Geometry: final body of the model. Coordinates: model frame, mm. Face numbers are marked on the shaded views. Give positions to 0.01 mm unless a question says otherwise; leave off trailing zeros. Write each loop counter-clockwise with the first axis right and the second up, starting at its lowest first coordinate (ties: lowest second). Pieces come first, ordered by that corner, then holes.
Q1. Mould query, pull axis Y, two halves, no side actions, for the marked faces 1 and 2. Classes: +Y half, -Y half, draft (parallel to the pull), parting line (faces both ways), or undercut.
Q2. Line query: line 1 (X direction, y = 81.5, z = -4.55); line 2 (X direction, y = 71.5, z = -4.15); line 3 (X direction, y = 40.5, z = -3.5). Output: solid intervals per line, ascending.
Q3. Section C-C (y = 42). Return the cut outline in (x, z), plus the area to 3 significant figures.
Q4. Section B-B (z = -1.2). Return the cut outline in (x, y).
Q5. Section A-A (x = 21). Return the cut outline in (y, z), plus the area to 3 significant figures.
Q6. Pin query (flat end, axial travel): pin 1 Ø2 at (y, z) = (83, -1.5) entering from -X; pin 2 Ø2.5 at (x, z) = (28.5, -1.5) entering from +Y. Return the tip coordinate at first contact, or that it passes through.
Q7. Section D-D (x = 30). State how many separate pieces and enclosed holes the cut face has, plus the area to 3 significant figures.
from build123d import *

# Parameters (mm, degrees)
SKETCH1_W          = 60
SKETCH1_H          = 100
SKETCH1_W_2        = 20
SKETCH1_H_2        = 40
EXTRUDE1_DEPTH     = 5
FILLET2_R          = 3
SHELL2_START       = -5
SHELL2_OUTLINE_W   = 55
SHELL2_OUTLINE_H   = 95
SHELL2_OUTLINE_W_2 = 25
SHELL2_OUTLINE_H_2 = 45
SHELL2_DEPTH       = 2.5
SHELL2_START_2     = 2.5
SHELL2_2_DEPTH     = 95
SHELL2_START_3     = 2
SHELL2_3_DEPTH     = 56


with BuildPart() as part:
    # Sketch1 → Extrude1 (new body)
    with BuildSketch(Plane.XY):
        with Locations((30, 50)):
            Rectangle(SKETCH1_W, SKETCH1_H)
        with Locations((30, 50)):
            Rectangle(SKETCH1_W_2, SKETCH1_H_2, mode=Mode.SUBTRACT)
        with BuildLine():
            Line((32.5, 80), (32.5, 90))
            ThreePointArc((32.5, 90), (30, 92.5), (27.5, 90))
            Line((27.5, 90), (27.5, 80))
            ThreePointArc((27.5, 80), (30, 77.5), (32.5, 80))
        make_face(mode=Mode.SUBTRACT)
        with BuildLine():
            Line((27.5, 10), (27.5, 20))
            ThreePointArc((27.5, 20), (30, 22.5), (32.5, 20))
            Line((32.5, 20), (32.5, 10))
            ThreePointArc((32.5, 10), (30, 7.5), (27.5, 10))
        make_face(mode=Mode.SUBTRACT)
    extrude(amount=-EXTRUDE1_DEPTH)

    # Fillet2
    fillet2_edges = [part.edges().sort_by_distance(p)[0] for p in [
        (30, 100, 0),
        (60, 50, 0),
        (30, 0, 0),
        (0, 50, 0),
    ]]
    fillet(fillet2_edges, radius=FILLET2_R)

    # Shell2: read off the stored shape, not the designer's step
    # Shell2 outline → Shell2 (cut)
    with BuildSketch(Plane.XY.offset(SHELL2_START)):
        with Locations((30, 50)):
            Rectangle(SHELL2_OUTLINE_W, SHELL2_OUTLINE_H)
        with BuildLine():
            Line((25, 10), (25, 20))
            ThreePointArc((25, 20), (30, 25), (35, 20))
            Line((35, 20), (35, 10))
            ThreePointArc((35, 10), (30, 5), (25, 10))
        make_face(mode=Mode.SUBTRACT)
        with Locations((30, 50)):
            Rectangle(SHELL2_OUTLINE_W_2, SHELL2_OUTLINE_H_2, mode=Mode.SUBTRACT)
        with BuildLine():
            ThreePointArc((35, 80), (30, 75), (25, 80))
            Line((25, 80), (25, 90))
            ThreePointArc((25, 90), (30, 95), (35, 90))
            Line((35, 90), (35, 80))
        make_face(mode=Mode.SUBTRACT)
    extrude(amount=SHELL2_DEPTH, mode=Mode.SUBTRACT)

    # Shell2 2 outline → Shell2 2 (add)
    with BuildSketch(Plane(origin=(0, 0, 0), x_dir=(1, 0, 0), z_dir=(0, 1, 0)).offset(SHELL2_START_2)):
        with BuildLine():
            Line((57.5, 2.5), (57.5, 3))
            ThreePointArc((57.5, 3), (57.353553391, 2.646446609), (57, 2.5))
            Line((57, 2.5), (57.5, 2.5))
        make_face()
        with BuildLine():
            Line((2.5, 2.5), (3, 2.5))
            ThreePointArc((3, 2.5), (2.646446609, 2.646446609), (2.5, 3))
            Line((2.5, 3), (2.5, 2.5))
        make_face()
    extrude(amount=SHELL2_2_DEPTH)

    # Shell2 3 outline → Shell2 3 (add)
    with BuildSketch(Plane.YZ.offset(SHELL2_START_3)):
        with BuildLine():
            ThreePointArc((2.5, -3), (2.646446609, -2.646446609), (3, -2.5))
            Line((3, -2.5), (2.5, -2.5))
            Line((2.5, -2.5), (2.5, -3))
        make_face()
        with BuildLine():
            ThreePointArc((97, -2.5), (97.353553391, -2.646446609), (97.5, -3))
            Line((97.5, -3), (97.5, -2.5))
            Line((97.5, -2.5), (97, -2.5))
        make_face()
    extrude(amount=SHELL2_3_DEPTH)


solid = part.part
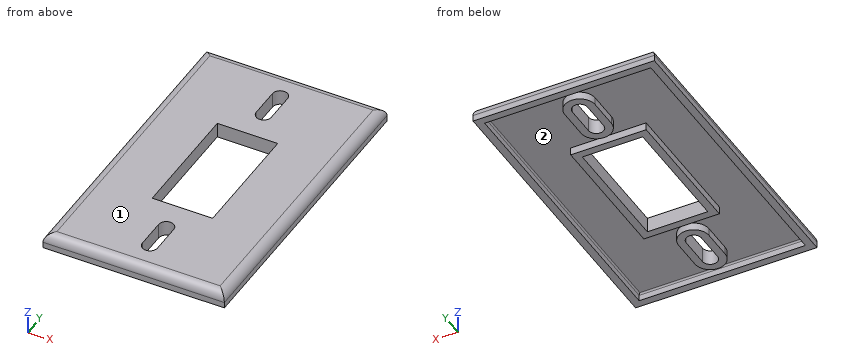
Computed:
1. face 1: draft
1. face 2: undercut
2. line 1: x = 0 to 2.5, 25 to 27.5, 32.5 to 35, 57.5 to 60
2. line 2: x = 0 to 2.5, 17.5 to 42.5, 57.5 to 60
2. line 3: x = 0 to 2.5, 17.5 to 20, 40 to 42.5, 57.5 to 60
3. outline: (0, -5) - (2.5, -5) - (2.5, -3) arc R0.5 cw to (3, -2.5) - (17.5, -2.5) - (17.5, -5) - (20, -5) - (20, 0) - (3, 0) arc R3 ccw to (0, -3) - close; (40, -5) - (42.5, -5) - (42.5, -2.5) - (57, -2.5) arc R0.5 cw to (57.5, -3) - (57.5, -5) - (60, -5) - (60, -3) arc R3 ccw to (57, 0) - (40, 0) - close
3. area: 121 mm2
4. outline: (0.6, 0.6) - (59.4, 0.6) - (59.4, 99.4) - (0.6, 99.4) - close; hole (20, 30) - (40, 30) - (40, 70) - (20, 70) - close; hole (27.5, 10) arc R2.5 ccw to (32.5, 10) - (32.5, 20) arc R2.5 ccw to (27.5, 20) - close; hole (27.5, 80) arc R2.5 ccw to (32.5, 80) - (32.5, 90) arc R2.5 ccw to (27.5, 90) - close
5. outline: (0, -5) - (2.5, -5) - (2.5, -3) arc R0.5 cw to (3, -2.5) - (27.5, -2.5) - (27.5, -5) - (30, -5) - (30, 0) - (3, 0) arc R3 ccw to (0, -3) - close; (70, -5) - (72.5, -5) - (72.5, -2.5) - (97, -2.5) arc R0.5 cw to (97.5, -3) - (97.5, -5) - (100, -5) - (100, -3) arc R3 ccw to (97, 0) - (70, 0) - close
5. area: 171 mm2
6. pin 1: stops at x = 0.04
6. pin 2: stops at y = 99.99
7. separate pieces: 4
7. enclosed holes: 0
7. area: 121 mm2
